Input: part model. Units: mm. Frame: model coordinates. Face numbers are marked on the shaded views. A direction names the side the tool comes from. Round coordinates to 2 decimals unless told otherwise and drop trailing zeros. Write each loop counter-clockwise with the first axis right and the second up, starting at its lowest first coordinate (ties: lowest second). Pieces come first, ordered by that corner, then holes. Notation, with made-up numbers: (69, 39) - (103, 39) arc R17 cw to (103, 69) - close; hole circle Ø11 at (27, 48.5). An arc over 180 degrees is marked (long way). One line per item, written item: value. Start each with the question number.
```python
from build123d import *

# Parameters (mm, degrees)
F1_DEPTH = 22.5
F3_DEPTH = 25
F7_R     = 5
F8_R     = 5
F9_R     = 2.5


with BuildPart() as f1:
    # F0 (on Front) → F1 (new body)
    with BuildSketch(Plane.XZ):
        with BuildLine():
            Line((0, 42), (0, 5))
            ThreePointArc((0, 5), (1.4644660941, 1.4644660941), (5, 0))
            Line((5, 0), (65, 0))
            ThreePointArc((65, 0), (68.5355339059, 1.4644660941), (70, 5))
            Line((70, 5), (70, 20))
            Line((70, 20), (60, 20))
            Line((60, 20), (60, 17))
            ThreePointArc((60, 17), (58.5355339059, 13.4644660941), (55, 12))
            Line((55, 12), (15, 12))
            ThreePointArc((15, 12), (11.4644660941, 13.4644660941), (10, 17))
            Line((10, 17), (10, 42))
            Line((10, 42), (0, 42))
        make_face()
    extrude(amount=F1_DEPTH)

    # F2 (on face) → F3 (cut)
    with BuildSketch(Plane.YZ.offset(10)):
        with BuildLine():
            ThreePointArc((-8.75, 29.5), (-9.482233047, 31.267766953), (-11.25, 32))
            Line((-11.25, 32), (-11.25, 27))
            ThreePointArc((-11.25, 27), (-9.482233047, 27.732233047), (-8.75, 29.5))
        make_face()
        with BuildLine():
            Line((-11.25, 27), (-11.25, 32))
            ThreePointArc((-11.25, 32), (-13.75, 29.5), (-11.25, 27))
        make_face()
    extrude(amount=-F3_DEPTH, mode=Mode.SUBTRACT)

    # F5 (on line) → F6 (revolve, cut)
    with BuildSketch(Plane(origin=(0, -11.25, 0), x_dir=(-1, 0, 0), z_dir=(0, 1, 0))):
        Polygon((-6.5, 32), (-10, 35.5), (-10, 32), align=None)
    revolve(axis=Axis((5, -11.25, 29.5), (-1, 0, 0)), mode=Mode.SUBTRACT)

    # F7
    f7_edges = [f1.edges().sort_by_distance(p)[0] for p in [
        (60, -11.25, 20),
    ]]
    fillet(f7_edges, radius=F7_R)

    # F8
    f8_edges = [f1.edges().sort_by_distance(p)[0] for p in [
        (70, -11.25, 20),
    ]]
    fillet(f8_edges, radius=F8_R)

    # F9
    f9_edges = [f1.edges().sort_by_distance(p)[0] for p in [
        (35, 0, 12),
        (35, -22.5, 12),
    ]]
    fillet(f9_edges, radius=F9_R)


solid = f1.part
```
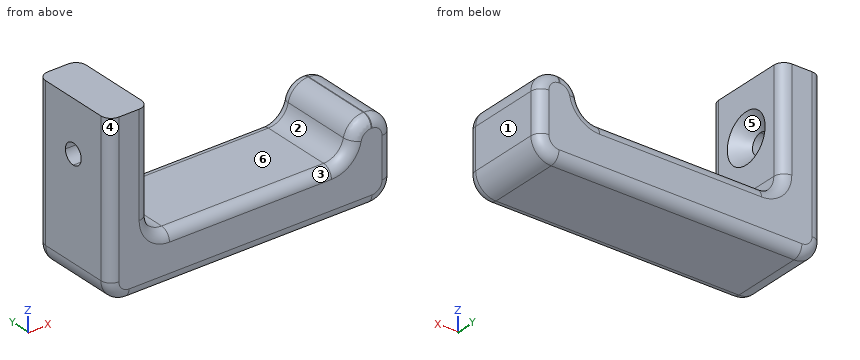
Q1. Material intervals for probe 1 along Z at (x, y) = (43.5, -5.75); probe 2 along X at (y, z) = (-17.25, 37); probe 3 along X at (y, z) = (-16, 19), sorted ascending. Write a range as from..to.
Q2. Contact query for flat-ended pins moving along their axis: pin 1 Ø9 at (x, y) = (38.5, -10.5) entering from +Z; pin 2 Ø1.5 at (y, z) = (-16.5, 25.5) entering from +X. Output: stop coordinate, or through.
Q3. Pull-direction query (Y, two-part tool) for the marked faces 4, 5 and 6; classes: pulls with the +Y half, pulls with the -Y half, needs draft (parallel to the pull), parting line crosses it, or undercut.
Q4. Access query for the marked faces 1, 2 and 3. Directions: +Z, -Z, +X, -X, +Y, -Y. A direction counts if a zero-diameter tool reaches every point of the face in a straight line with its end or side. Return the directions, or none.
Q5. Cut plane A-A, the plane x = 32.5. Output: boundary loops of the cut face in (y, z).
A:
1. probe 1: z = 0..12
1. probe 2: x = 0..10
1. probe 3: x = 0..10, 61.8..68
2. pin 1: stops at z = 12
2. pin 2: stops at x = 10
3. face 4: pulls with the -Y half
3. face 5: undercut
3. face 6: needs draft
4. face 1: +Z, -Z, +X, +Y, -Y
4. face 2: +Z, +Y, -Y
4. face 3: +Z, -Y
5. outline: (-22.5, 2.5) arc R2.5 ccw to (-20, 0) - (-2.5, 0) arc R2.5 ccw to (0, 2.5) - (0, 9.5) arc R2.5 ccw to (-2.5, 12) - (-20, 12) arc R2.5 ccw to (-22.5, 9.5) - close
